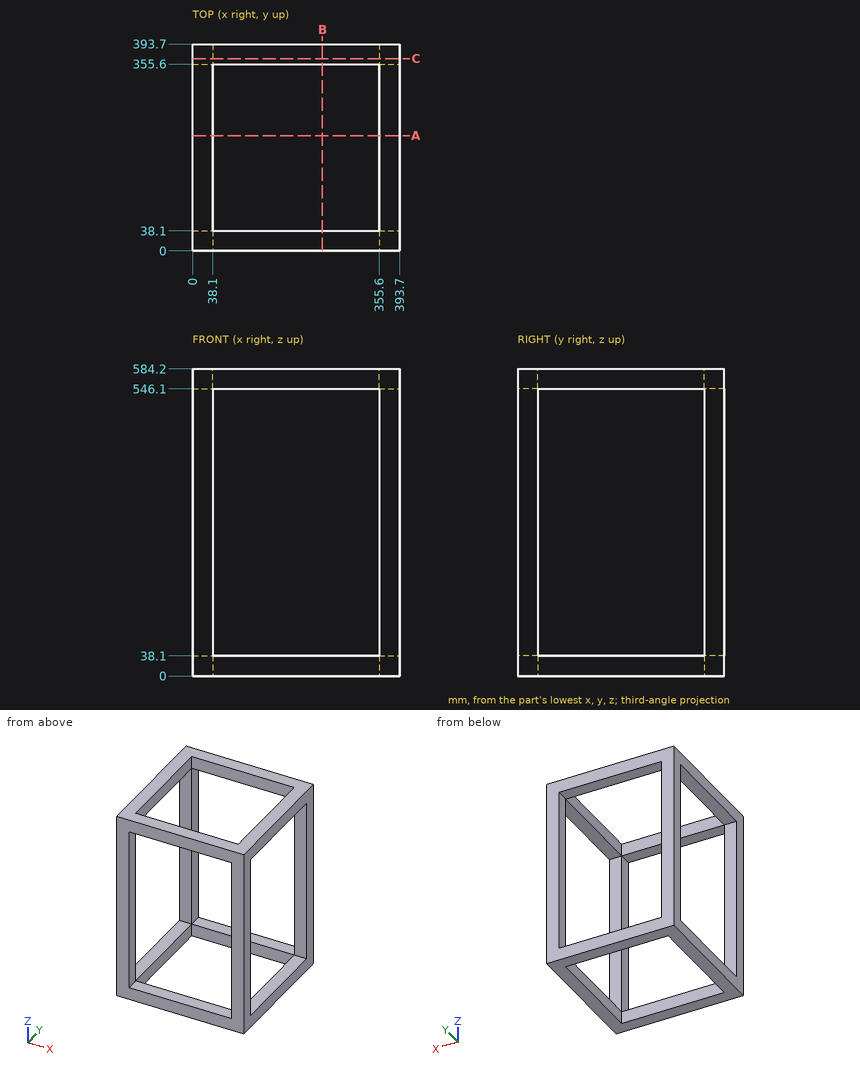
Can you work these out from the drawing? Everything is in mm from the part's minimum corner. Coordinates: 2 decimals unless noted, no trailing zeros. Write each loop counter-clockwise with the first axis right and the second up, starting at its lowest first coordinate (ties: lowest second). Pieces come first, ordered by that corner, then holes. Notation, with made-up numbers: (34, 57) -> (57, 57) arc R13 ccw to (57, 74) -> close; hole circle Ø10 at (-22.75, -26.75). An arc over 180 degrees is marked (long way). Write each question's results on one line, items separated by ' | '. Start each with the question number.
Q1. I'm going to push a flat-ended pin straight in: pin 1 (11.5 mm diameter, centred on x = 369.5, y = 202.5, fed in from -Z). Where does the tip first touch, or does it pass through?
Q2. If I drill on probe 1 along Y at (x, z) = (376, 534.5); probe 2 along Z at (x, y) = (125.5, 24), over which ranges is the centre line in solid material (lowest first)?
Q3. Imagine slicing it at A-A (y = 219.5). Write out the boundary of the cut face in (x, z).
Q4. Imagine slicing it at C-C (y = 366). Write out the boundary of the cut face in (x, z), then the cut area to 3 significant figures.
Taken from the geometry:
1) pin 1: stops at z = 0
2) probe 1: y = 0 to 38.1, 355.6 to 393.7 | probe 2: z = 0 to 38.1, 546.1 to 584.2
3) outline: (0, 0) -> (38.1, 0) -> (38.1, 38.1) -> (0, 38.1) -> close; (0, 546.1) -> (38.1, 546.1) -> (38.1, 584.2) -> (0, 584.2) -> close; (355.6, 0) -> (393.7, 0) -> (393.7, 38.1) -> (355.6, 38.1) -> close; (355.6, 546.1) -> (393.7, 546.1) -> (393.7, 584.2) -> (355.6, 584.2) -> close
4) outline: (0, 0) -> (393.7, 0) -> (393.7, 584.2) -> (0, 584.2) -> close; hole (38.1, 38.1) -> (355.6, 38.1) -> (355.6, 546.1) -> (38.1, 546.1) -> close | area: 68,700 mm^2
